Can you work these out from the drawing? Everything is in mm from the part's minimum corner. A direction names the side the tool comes from. Give positions to 0.01 mm unless a question says otherwise; leave off trailing zeros. Write each loop counter-clockwise with the first axis right and the second up, starting at its lowest first coordinate (ties: lowest second). Pieces come first, ordered by that corner, then holes. Notation, with made-up numbers: (25, -17) -> (78, -17) arc R4 ccw to (78, -10) -> close; hole circle Ø8 at (65.25, -1). An arc over 180 degrees is marked (long way). Return JSON: item names as keys, results as strings.
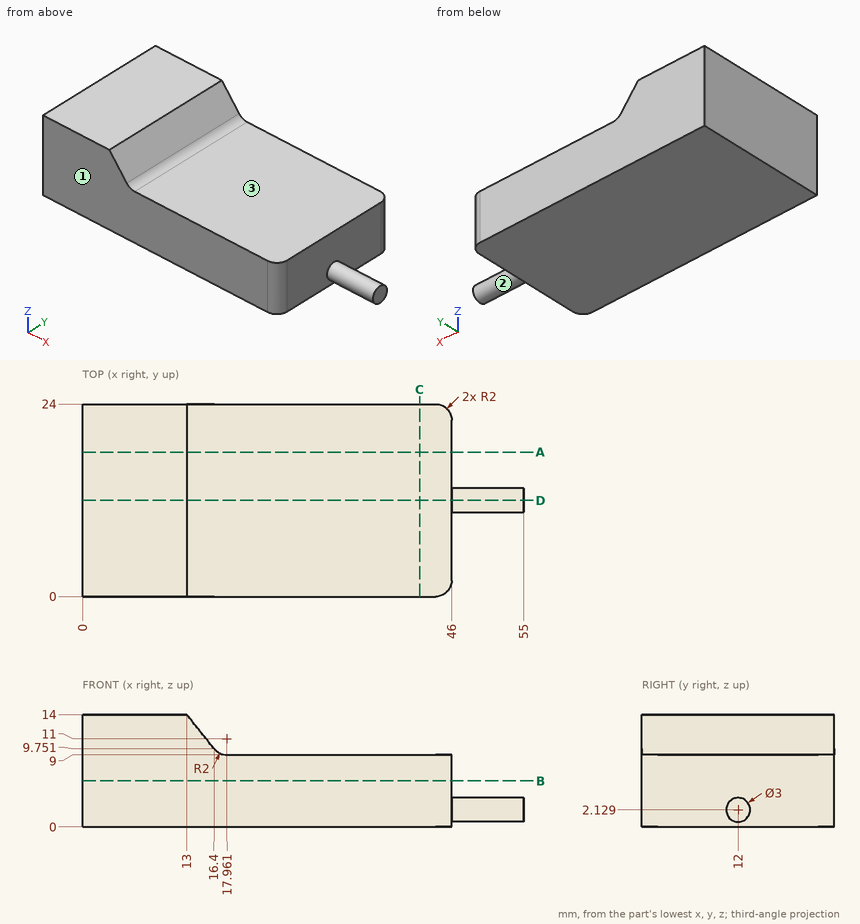
1. Suppose I cut it at A-A, the plane y = 18. List the corners of the cut face in (x, z) for me, and give its area (3 significant figures).
Taken from the geometry:
{"outline": "(0, 0) -> (46, 0) -> (46, 9) -> (17.96, 9) arc R2 cw to (16.4, 9.75) -> (13, 14) -> (0, 14) -> close", "area": "489 mm²"}
2. Suppose I cut it at D-D, the plane y = 12. List the corners of the cut face in (x, z) for me.
Taken from the geometry:
{"outline": "(0, 0) -> (46, 0) -> (46, 0.63) -> (55, 0.63) -> (55, 3.63) -> (46, 3.63) -> (46, 9) -> (17.96, 9) arc R2 cw to (16.4, 9.75) -> (13, 14) -> (0, 14) -> close"}
3. Suppose I cut it at C-C, the plane x = 42. List the corners of the cut face in (y, z) for me.
Taken from the geometry:
{"outline": "(0, 0) -> (24, 0) -> (24, 9) -> (0, 9) -> close"}
4. Suppose I cut it at B-B, the plane z = 5.75. List the corners of the cut face in (x, y) for me, and give its area (3 significant figures).
Taken from the geometry:
{"outline": "(0, 0) -> (44, 0) arc R2 ccw to (46, 2) -> (46, 22) arc R2 ccw to (44, 24) -> (0, 24) -> close", "area": "1,100 mm²"}
5. Which directions (+Z, -Z, +X, -X, +Y, -Y) give clear straight access to the entire face, cutting with the end or side of a thin tool? Please do the marked faces 1, 2 and 3.
Taken from the geometry:
{"face 1": "+Z, -Z, +X, -X, -Y", "face 2": "+X", "face 3": "+Z, +X, +Y, -Y"}
6. If I drill on line 1 (Z direction, x = 26.5, y = 17.75); line 2 (X direction, y = 16, z = 5.75); line 3 (X direction, y = 15.5, z = 13.25), over which ranges is the centre line in solid material (lowest first)? Write a range as [from, to].
Taken from the geometry:
{"line 1": "z = [0, 9]", "line 2": "x = [0, 46]", "line 3": "x = [0, 13.6]"}
7. For pin 1 Ø5 at (x, z) = (35.5, 12) entering from +Y (1 decimal); pin 2 Ø5 at (x, y) = (33, 16) entering from +Z, each with a flat end and sliding along its axis, tell me the tip position at first contact or that it passes through.
Taken from the geometry:
{"pin 1": "passes through", "pin 2": "stops at z = 9"}
